```python
from build123d import *

# Parameters (mm, degrees)
SKETCH1_R                    = 12.5
SKETCH1_R_2                  = 6
BOSS_EXTRUDE1_DEPTH          = 24
SKETCH1_2_R                  = 6
BOSS_EXTRUDE2_DEPTH          = 480
SKETCH1_4_R                  = 12.5
BOSS_EXTRUDE3_DEPTH          = 48
M8_START                     = -17.5
M8_CLEARANCE_HOLE1_OUTLINE_R = 5
M8_CLEARANCE_HOLE1_DEPTH     = 35
SKETCH4_R                    = 4
CUT_EXTRUDE1_DEPTH           = 30


# Read off the part's stored shape, not the designer's step: M8 Clearance Hole1
with BuildPart() as part:
    # Sketch1 → Boss-Extrude1 (new body)
    # profile 1 of 2: a face of its own
    with BuildSketch(Plane.XY):
        Polygon((18.05, 17.5), (18.05, 25.5), (-18.05, 25.5), (-18.05, 17.5), (-35, 17.5), (-35, -17.5), (35, -17.5), (35, 17.5), align=None)
        with Locations((0, 7.5)):
            Circle(SKETCH1_R, mode=Mode.SUBTRACT)
    # profile 2 of 2: a face of its own
    with BuildSketch(Plane.XY):
        with Locations((0, 7.5)):
            Circle(SKETCH1_R)
        with Locations((0, 7.5)):
            Circle(SKETCH1_R_2, mode=Mode.SUBTRACT)
    extrude(amount=BOSS_EXTRUDE1_DEPTH)

    # Sketch1<2> → Boss-Extrude2 (add)
    with BuildSketch(Plane.XY):
        with Locations((0, 7.5)):
            Circle(SKETCH1_2_R)
    extrude(amount=BOSS_EXTRUDE2_DEPTH)

    # Sketch1<4> → Boss-Extrude3 (add)
    with BuildSketch(Plane.XY):
        with Locations((0, 7.5)):
            Circle(SKETCH1_4_R)
    extrude(amount=-BOSS_EXTRUDE3_DEPTH)

    # M8 Clearance Hole1 outline → M8 Clearance Hole1 (cut)
    with BuildSketch(Plane(origin=(0, 0, 0), x_dir=(1, 0, 0), z_dir=(0, 1, 0)).offset(M8_START)):
        with Locations((25.75, -12)):
            Circle(M8_CLEARANCE_HOLE1_OUTLINE_R)
        with Locations((-25.75, -12)):
            Circle(M8_CLEARANCE_HOLE1_OUTLINE_R)
    extrude(amount=M8_CLEARANCE_HOLE1_DEPTH, mode=Mode.SUBTRACT)

    # Sketch4 → Cut-Extrude1 (cut)
    with BuildSketch(Plane(origin=(0, 0, -48), x_dir=(-1, 0, 0), z_dir=(0, 0, -1))):
        with Locations((0, 7.5)):
            Circle(SKETCH4_R)
    extrude(amount=-CUT_EXTRUDE1_DEPTH, mode=Mode.SUBTRACT)


solid = part.part
```
The listing builds one solid part. Answer for the finished solid, in the listing's coordinates (mm). A direction names the side the tool comes from. Give positions to 0.01 mm unless a question says otherwise; leave off trailing zeros. Loops run counter-clockwise (first coordinate to the right, second up) from the corner with the lowest first, then second, coordinate; pieces in that order, holes last. Notation, with made-up numbers: (-6, 28) - (13, 28) arc R20 ccw to (13, 35) - close; hole circle Ø6 at (71, -24). An arc over 180 degrees is marked (long way). Answer as CSV lines item,"result". Start each with the question number.
Item 1: A cutting plane is placed at C-C on z = 108. Determine the outline of the cut face in (x, y), then the cut area to 3 significant figures.
Item 2: A cutting plane is placed at A-A on z = 12. Determine the outline of the cut face in (x, y), then the cut area to 3 significant figures.
Item 3: For faces 1 (the face through (-5.994, 7.764, 248.808)), 2 (the face through (35, 0, 12)), 3 (the face through (-2.71, -4.703, -23.664)), 4 (the face through (30, 17.5, 9)), determine the directions among +Z, -Z, +X, -X, +Y, -Y from which every point of the face is accessible in a straight line to the end or side of a thin tool.
Item 4: The mould has two halves that part along Z. Classify faces 5 (the face through (-30, 17.5, 9)), 6 (the face through (-30.745, -0.245, 11.78)), 7 (the face through (0, 0, 24)): +Z half, -Z half, draft (parallel to the pull), parting line (faces both ways), or undercut.
Item 5: Find the intervals of material crossed by line 1 (X direction, y = 7, z = 12); line 2 (Y direction, x = 0, z = -39.5); line 3 (Z direction, x = 11, y = -11.5), in increasing order. Write a range as from..to.
Item 6: Each of these flat-tipped pins is pushed along its axis until it touches: pin 1 (12 mm diameter, centred on x = 0, z = 220, fed in from -Y); pin 2 (4 mm diameter, centred on y = 21.5, z = 11.5, fed in from +X); pin 3 (4 mm diameter, centred on y = 23.5, z = 10.5, fed in from -X); pin 4 (18.5 mm diameter, centred on x = 22.5, z = 15.5, fed in from +Y). Where does it stop, or does it pass through?
Item 7: A cutting plane is placed at B-B on x = -25.75. Determine the outline of the cut face in (y, z).
Found:
1,outline,"circle Ø12 at (0, 7.5)"
1,area,"113 mm^2"
2,outline,"(-35, -17.5) - (-30.75, -17.5) - (-30.75, 17.5) - (-35, 17.5) - close; (-20.75, -17.5) - (20.75, -17.5) - (20.75, 17.5) - (18.05, 17.5) - (18.05, 25.5) - (-18.05, 25.5) - (-18.05, 17.5) - (-20.75, 17.5) - close; (30.75, -17.5) - (35, -17.5) - (35, 17.5) - (30.75, 17.5) - close"
2,area,"2,040 mm^2"
3,face 1,"+Z"
3,face 2,"+Z, -Z, +X, +Y, -Y"
3,face 3,"-Z"
3,face 4,"+Z, -Z, +X, +Y"
4,face 5,"draft"
4,face 6,"undercut"
4,face 7,"+Z half"
5,line 1,"x = -35..-30.75, -20.75..20.75, 30.75..35"
5,line 2,"y = -5..3.5, 11.5..20"
5,line 3,"z = 0..24"
6,pin 1,"stops at y = 1.5"
6,pin 2,"stops at x = 18.05"
6,pin 3,"stops at x = -18.05"
6,pin 4,"stops at y = 25.5"
7,outline,"(-17.5, 0) - (17.5, 0) - (17.5, 7) - (-17.5, 7) - close; (-17.5, 17) - (17.5, 17) - (17.5, 24) - (-17.5, 24) - close"
